Geometry: final body of the model. Coordinates: model frame, mm. A direction names the side the tool comes from. Coordinates: 2 decimals unless noted, no trailing zeros. Write each loop counter-clockwise with the first axis right and the second up, starting at its lowest first coordinate (ties: lowest second). Pieces come first, ordered by that corner, then holes. Notation, with made-up numbers: (-35.5, -27.75) -> (6.5, -27.75) arc R9 ccw to (6.5, -12.75) -> close; hole circle Ø3 at (73, -18). An arc over 180 degrees is marked (long way). Answer as a JSON object with one key per item and string values. Group by question number.
```python
from build123d import *

# Parameters (mm, degrees)
F0_R     = 1.25
F1_DEPTH = 2.5


with BuildPart() as f1:
    # F0 (on Top) → F1 (new body)
    with BuildSketch(Plane.XY):
        with BuildLine():
            Line((0, -4), (0, 0))
            Line((0, 0), (-0.0945953157, 0))
            ThreePointArc((-0.0945953157, 0), (-1.7241340654, -4), (-0.0945953157, -8))
            Line((-0.0945953157, -8), (0, -8))
            Line((0, -8), (0, -4))
        make_face()
        with BuildLine():
            Line((-0.0945953157, 0), (0, 0))
            Line((0, 0), (0, -4))
            Line((0, -4), (0, -8))
            Line((0, -8), (-0.0945953157, -8))
            ThreePointArc((-0.0945953157, -8), (6.159594669, -9.3011189069), (9.7241340654, -4))
            ThreePointArc((9.7241340654, -4), (6.159594669, 1.3011189069), (-0.0945953157, 0))
        make_face()
        with BuildLine():
            ThreePointArc((5.25, -4), (4, -5.25), (2.75, -4))
            ThreePointArc((2.75, -4), (4, -2.75), (5.25, -4))
        make_face(mode=Mode.SUBTRACT)
        with BuildLine():
            ThreePointArc((-0.0945953157, -8), (-1.7241340654, -4), (-0.0945953157, 0))
            Line((-0.0945953157, 0), (-27, 0))
            Line((-27, 0), (-27, -0.058367438))
            ThreePointArc((-27, -0.058367438), (-25.8038763073, -1.870031497), (-25.3842660984, -4))
            ThreePointArc((-25.3842660984, -4), (-25.8038763073, -6.129968503), (-27, -7.941632562))
            Line((-27, -7.941632562), (-27, -8))
            Line((-27, -8), (-0.0945953157, -8))
        make_face()
        with BuildLine():
            ThreePointArc((-25.3842660984, -4), (-25.8038763073, -1.870031497), (-27, -0.058367438))
            Line((-27, -0.058367438), (-27, -4))
            Line((-27, -4), (-27, -7.941632562))
            ThreePointArc((-27, -7.941632562), (-25.8038763073, -6.129968503), (-25.3842660984, -4))
        make_face()
        with BuildLine():
            Line((-27, -4), (-27, -0.058367438))
            ThreePointArc((-27, -0.058367438), (-36.6157339016, -4), (-27, -7.941632562))
            Line((-27, -7.941632562), (-27, -4))
        make_face()
        with Locations((-31, -4)):
            Circle(F0_R, mode=Mode.SUBTRACT)
    extrude(amount=F1_DEPTH)


solid = f1.part
```
Item 1: Section D-D on x = -1. Output: boundary loops of the cut face in (y, z), then the cut area to 3 significant figures.
Item 2: Set-up query: faces 4 (the flat face through (-13, 0, 1)), 5 (the cylindrical face through (-29.845, -4.479, 1.232)). Return all of +Z, -Z, +X, -X, +Y, -Y with unobstructed straight access to the full face (end or side cutting, diameter ignored); none if empty.
Item 3: Ray query, L1, parallel to Y at x = -31, z = 1.3; L2, parallel to Y at x = 4, z = 1.75; L3, parallel to X at y = -4.5, z = 0.7. Return the intervals inside material, ascending. Write a range as [from, to].
Item 4: Contact query for flat-ended pins moving along their axis: pin 1 (6 mm diameter, centred on x = -16, y = -8.5, fed in from +Z); pin 2 (1.5 mm diameter, centred on x = 4, y = -4, fed in from +Z). Output: stop coordinate, or through.
Item 5: Section B-B on z = 0.5. Output: boundary loops of the cut face in (x, y), then the cut area to 3 significant figures.
Item 6: Section C-C on y = -8.5. Output: boundary loops of the cut face in (x, z), then the cut area to 3 significant figures.
Item 7: Mould query, pull axis X, two halves, no side actions, for faces 1 (the flat face through (-14, -8, 1)), 2 (the cylindrical face through (4.27, -5.22, 1.23)), 3 (the flat face through (-14, -4, 2.5)). Classes: +X half, -X half, draft (parallel to the pull), parting line (faces both ways), or undercut.
Item 8: Section A-A on x = 4. Output: boundary loops of the cut face in (y, z), then the cut area to 3 significant figures.
Answer sheet:
{
 "1": {"outline": "(-8, 0) -> (0, 0) -> (0, 2.5) -> (-8, 2.5) -> close", "area": "20.0 mm^2"},
 "2": {"face 4": "+Z, -Z, +Y", "face 5": "+Z, -Z"},
 "3": {"L1": "y = [-9.62, -5.25], [-2.75, 1.62]", "L2": "y = [-9.72, -5.25], [-2.75, 1.72]", "L3": "x = [-36.59, -32.15], [-29.85, 2.85], [5.15, 9.7]"},
 "4": {"pin 1": "stops at z = 2.5", "pin 2": "passes through"},
 "5": {"outline": "(-27, -8) -> (-0.09, -8) arc R5.72 ccw (long way) to (-0.09, 0) -> (-27, 0) -> (-27, -0.06) arc R5.62 ccw (long way) to (-27, -7.94) -> close; hole circle Ø2.5 at (-31, -4); hole circle Ø2.5 at (4, -4)", "area": "390 mm^2"},
 "6": {"outline": "(-34.36, 0) -> (-27.64, 0) -> (-27.64, 2.5) -> (-34.36, 2.5) -> close; (0.46, 0) -> (7.54, 0) -> (7.54, 2.5) -> (0.46, 2.5) -> close", "area": "34.5 mm^2"},
 "7": {"face 1": "undercut", "face 2": "undercut", "face 3": "draft"},
 "8": {"outline": "(-9.72, 0) -> (-5.25, 0) -> (-5.25, 2.5) -> (-9.72, 2.5) -> close; (-2.75, 0) -> (1.72, 0) -> (1.72, 2.5) -> (-2.75, 2.5) -> close", "area": "22.4 mm^2"}
}
